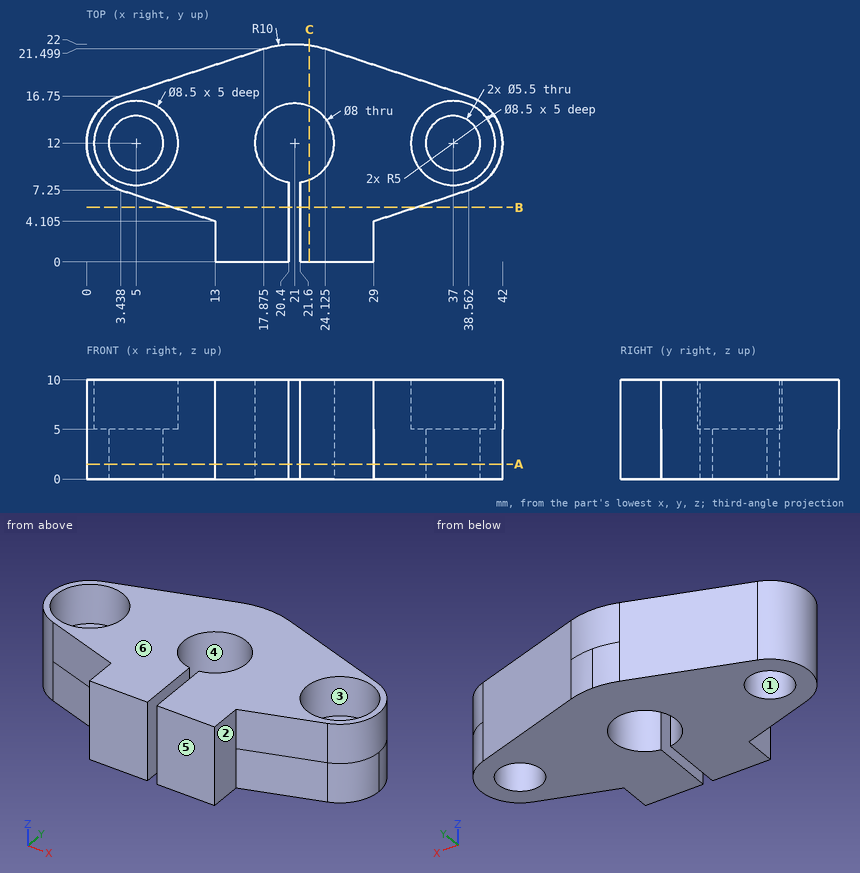
Check sheet for the drawn part. Datum: minimum x, y, z corner. Units: mm. A direction names the side the tool comes from. Coordinates: 2 decimals unless noted, no trailing zeros. Order: outer loops, then holes, each group sorted by start corner. A loop starts at its lowest first (then second) coordinate and runs counter-clockwise, first axis right, second up. Notation, with made-up numbers: (81.25, -9) - (122.25, -9) arc R16 cw to (122.25, 13) - close; hole circle Ø6 at (75, 3.25). An arc over 180 degrees is marked (long way). Return JSON: item names as keys, results as strings.
(1) Mould release check, pull along Y, two halves, no side actions. Record for the marked faces 4, 5 and 6: pulls with the +Y half, pulls with the -Y half, needs draft (parallel to the pull), parting line crosses it, or undercut.
Filled sheet:
{"face 4": "undercut", "face 5": "pulls with the -Y half", "face 6": "needs draft"}
(2) Thickness scan on line 1 along X through (y, z) = (12.5, 6.25) (1 decimal); line 2 along X through (y, z) = (10.5, 7.5) (1 decimal); line 3 along X through (y, z) = (2.5, 6.5). Record the ranges inside material, lowest first.
Filled sheet:
{"line 1": "x = 0 to 0.8, 9.2 to 17, 25 to 32.8, 41.2 to 42", "line 2": "x = 0.2 to 1, 9 to 17.3, 24.7 to 33, 41 to 41.8", "line 3": "x = 13 to 20.4, 21.6 to 29"}
(3) Section check A-A, the plane z = 1.5. Give the number of separate pieces and of enclosed holes in the cut face.
Filled sheet:
{"separate pieces": "1", "enclosed holes": "2"}
(4) Section check B-B, the plane y = 5.5. Record the cut outline in (x, z).
Filled sheet:
{"outline": "(8.76, 0) - (20.4, 0) - (20.4, 10) - (8.76, 10) - close; (21.6, 0) - (33.24, 0) - (33.24, 10) - (21.6, 10) - close"}
(5) Section check C-C, the plane x = 22.5. Record the cut outline in (y, z), and give its area (3 significant figures).
Filled sheet:
{"outline": "(0, 0) - (8.29, 0) - (8.29, 10) - (0, 10) - close; (15.71, 0) - (21.89, 0) - (21.89, 10) - (15.71, 10) - close", "area": "145 mm^2"}
(6) Go/stop test with flat-tipped pins: pin 1 (5 mm diameter, centred on x = 17, y = 6, fed in from -Z); pin 2 (2.5 mm diameter, centred on x = 4, y = 12, fed in from +Z); pin 3 (1 mm diameter, centred on y = 13, z = 8.5, fed in from -X) (1 decimal); pin 4 (3 mm diameter, centred on y = 15, z = 6.5, fed in from -X). Record where each tip stops, or that it passes through.
Filled sheet:
{"pin 1": "stops at z = 0", "pin 2": "passes through", "pin 3": "stops at x = 0", "pin 4": "stops at x = 0.23"}
(7) Access from +Z, -Z, +X, -X, +Y, -Y to the whole of each face (thin tool, end or side, straight path). Record for the marked faces 1, 2 and 3.
Filled sheet:
{"face 1": "+Z, -Z", "face 2": "+Z, -Z, +X, -Y", "face 3": "+Z"}
